Autodesk Inventor part; units mm, degrees
ref_plane "YZ Plane" through (0, 0, 0) normal (1, 0, 0) x (0, 1, 0)
ref_plane "XZ Plane" through (0, 0, 0) normal (0, 1, 0) x (-1, 0, 0)
ref_plane "XY Plane" through (0, 0, 0) normal (0, 0, 1) x (1, 0, 0)
sketch "Sketch1" plane through (0, 0, 0) normal (0, 0, 1) x (1, 0, 0)
  line L0 (0, 0) -> (164.5, 0)
  line L1 (164.5, 0) -> (164.5, 10)
  line L2 (164.5, 10) -> (0, 10)
  line L3 (0, 10) -> (0, 0)
  circle A0 centre (57, 5) radius 1.6
  circle A1 centre (99, 5) radius 1.6
  circle A2 centre (159.5, 5) radius 1.6
  circle A3 centre (147, 5) radius 1.6
  circle A4 centre (15, 5) radius 1.6
  circle A5 centre (5, 5) radius 1.6
  dimension "d1" = 10
  dimension "d2" = 90
  dimension "d4" = 3.2
  dimension "d6" = 3.2
  dimension "d7" = 3.2
  dimension "d8" = 42
  dimension "d9" = 60.5
  dimension "d26" = 3.2
  dimension "d27" = 48
  dimension "d28" = 3.2
  dimension "d29" = 42
  dimension "d32" = 15
  dimension "d33" = 5
  dimension "d61" = 3.2
  dimension "d62" = 10
  dimension "d63" = 12.5
ref_plane "Work Plane2" through (0, 0, 0) normal (0, -1, 0) x (1, 0, 0)
sketch "Sketch2" plane through (0, 0, 0) normal (0, -1, 0) x (1, 0, 0)
  circle A0 centre (52, 7) radius 1.6
  circle A1 centre (125, 7) radius 1.6
  circle A2 centre (88.5, 7) radius 1.6
  point P0 (0, 0)
  dimension "d13" = 3.2
  dimension "d15" = 3.2
  dimension "d17" = 3.2
  dimension "d18" = 36.5
  dimension "d64" = 52
  dimension "d65" = 36.5
ref_plane "Work Plane1" through (0, 0, 11) normal (0, 0, 1) x (1, 0, 0)
extrude "klocek" add sketch "Sketch1" along normal blind 11
ref_plane "Work Plane3" through (0, 0, 0) normal (0, -1, 0) x (1, 0, 0)
extrude "prowadzenie osi" cut sketch "Sketch2" against normal up to next
ref_plane "Work Plane4" through (0, 0, 0) normal (0, -1, 0) x (1, 0, 0)
sketch "Sketch7" plane through (0, 0, 0) normal (0, -1, 0) x (1, 0, 0)
  line L0 (0, 11) -> (0, 0)
  line L1 (0, 11) -> (164.5, 11)
  line L2 (0, 11) -> (40, 11)
  line L3 (40, 11) -> (0, 0)
  point P0 (0, -1.8333)
  dimension "d86" = 11
  dimension "d87" = 40
sketch "Sketch8" plane through (0, 0, 0) normal (0, -1, 0) x (1, 0, 0)
  line L0 (164.5, 0) -> (164.5, 11)
  line L1 (164.5, 11) -> (164.5, 3)
  line L2 (164.5, 11) -> (0, 11)
  line L3 (164.5, 11) -> (134.5, 11)
  line L4 (134.5, 11) -> (164.5, 3)
  point P0 (0, 0)
  point P1 (40.8333, 11)
  dimension "d80" = 8
  dimension "d81" = 30
extrude "przedni skos" cut sketch "Sketch7" against normal up to next
extrude "tylni skos" cut sketch "Sketch8" against normal up to next
ref_plane "Work Plane7" through (0, 0, 11) normal (0, 0, 1) x (1, 0, 0)
sketch "Sketch5" plane through (0, 0, 11) normal (0, 0, 1) x (1, 0, 0)
  circle A0 centre (99, 5) radius 1.6
  line L0 (95.5936, 5) -> (97.2968, 7.95)
  line L1 (97.2968, 7.95) -> (100.7032, 7.95)
  line L2 (100.7032, 7.95) -> (102.4064, 5)
  line L3 (102.4064, 5) -> (100.7032, 2.05)
  line L4 (100.7032, 2.05) -> (97.2968, 2.05)
  line L5 (97.2968, 2.05) -> (95.5936, 5)
  circle A1 centre (57, 5) radius 1.6
  line L6 (60.4064, 5) -> (58.7032, 2.05)
  line L7 (58.7032, 2.05) -> (55.2968, 2.05)
  line L8 (55.2968, 2.05) -> (53.5936, 5)
  line L9 (53.5936, 5) -> (55.2968, 7.95)
  line L10 (55.2968, 7.95) -> (58.7032, 7.95)
  line L11 (58.7032, 7.95) -> (60.4064, 5)
  point P0 (119.5, 5)
  dimension "d98" = 5.9
  dimension "d100" = 5.9
extrude "hex insert middle" cut sketch "Sketch5" against normal blind 3
ref_plane "Work Plane6" through (0, 0, 11) normal (0, 0, 1) x (1, 0, 0)
sketch "Sketch9" plane through (0, 0, 11) normal (0, 0, 1) x (1, 0, 0)
  circle A0 centre (147, 5) radius 1.6
  line L0 (150.4064, 5) -> (148.7032, 2.05)
  line L1 (148.7032, 2.05) -> (145.2968, 2.05)
  line L2 (145.2968, 2.05) -> (143.5936, 5)
  line L3 (143.5936, 5) -> (145.2968, 7.95)
  line L4 (145.2968, 7.95) -> (148.7032, 7.95)
  line L5 (148.7032, 7.95) -> (150.4064, 5)
  point P0 (0, 0)
  point P1 (153, 5)
  dimension "d99" = 5.9
extrude "hex insert rear 1" cut sketch "Sketch9" against normal blind 6
ref_plane "Work Plane5" through (0, 0, 11) normal (0, 0, 1) x (1, 0, 0)
sketch "Sketch10" plane through (0, 0, 11) normal (0, 0, 1) x (1, 0, 0)
  circle A0 centre (159.5, 5) radius 1.6
  line L0 (162.9064, 5) -> (161.2032, 2.05)
  line L1 (161.2032, 2.05) -> (157.7968, 2.05)
  line L2 (157.7968, 2.05) -> (156.0936, 5)
  line L3 (156.0936, 5) -> (157.7968, 7.95)
  line L4 (157.7968, 7.95) -> (161.2032, 7.95)
  line L5 (161.2032, 7.95) -> (162.9064, 5)
  point P0 (0, 0)
  dimension "d101" = 5.9
extrude "hex insert rear 2" cut sketch "Sketch10" against normal blind 8.5
sketch "Sketch13" plane through (0, 0, 11) normal (0, 0, 1) x (1, 0, 0)
  circle A0 centre (5, 5) radius 1.6
  line L0 (8.4064, 5) -> (6.7032, 2.05)
  line L1 (6.7032, 2.05) -> (3.2968, 2.05)
  line L2 (3.2968, 2.05) -> (1.5936, 5)
  line L3 (1.5936, 5) -> (3.2968, 7.95)
  line L4 (3.2968, 7.95) -> (6.7032, 7.95)
  line L5 (6.7032, 7.95) -> (8.4064, 5)
  point P0 (0, 0)
  dimension "d90" = 5.9
extrude "hex insert front 1" cut sketch "Sketch13" against normal through all
sketch "Sketch16" plane through (0, 0, 11) normal (0, 0, 1) x (1, 0, 0)
  circle A0 centre (15, 5) radius 1.6
  line L0 (18.4064, 5) -> (16.7032, 2.05)
  line L1 (16.7032, 2.05) -> (13.2968, 2.05)
  line L2 (13.2968, 2.05) -> (11.5936, 5)
  line L3 (11.5936, 5) -> (13.2968, 7.95)
  line L4 (13.2968, 7.95) -> (16.7032, 7.95)
  line L5 (16.7032, 7.95) -> (18.4064, 5)
  point P0 (0, 0)
  dimension "d93" = 5.9
extrude "hex insert front 2" cut sketch "Sketch16" against normal blind 9
sketch "Sketch17" plane through (0, 0, 0) normal (0, 0, -1) x (-1, 0, 0)
  line L0 (0, 10) -> (0, 0)
  line L1 (0, 0) -> (-3.2968, 0)
  line L2 (-3.2968, 0) -> (-3.2968, 10.0042)
  line L3 (-3.2968, 10.0042) -> (0, 10.0042)
  line L4 (0, 10.0042) -> (0, 0)
extrude "Extrusion20" cut sketch "Sketch17" against normal up to next
sketch "Sketch18" plane through (40, 0, 11) normal (0, -1, 0) x (1, 0, 0)
  line L0 (9.5, 0) -> (9.5, -2)
  line L1 (9.5, -2) -> (-3.5, -2)
  line L2 (-3.5, -2) -> (-3.5, 0)
  line L3 (-3.5, 0) -> (9.5, 0)
  line L4 (94.5, 0) -> (0, 0)
  circle A0 centre (12, -4) radius 1.6
  line L5 (-36.7032, -11) -> (124.5, -11)
  point P0 (-40, -11)
  dimension "d102" = 2
  dimension "d103" = 13
  dimension "d104" = 2.5
extrude "Extrusion21" cut sketch "Sketch18" against normal blind 8 contours L0 L1 L2 L3
properties part number "wheel_support_v2"
Geometry check sheet. Reference: the model listing, model coordinates, mm. A direction names the side the tool comes from. Round coordinates to 2 decimals unless told otherwise and drop trailing zeros. Loops run counter-clockwise (first coordinate to the right, second up) from the corner with the lowest first, then second, coordinate; pieces in that order, holes last. Notation, with made-up numbers: M 6,-24 L 51,-24 A10 cw 51,-9 Z; hole C 34,23 d7. An arc over 180 degrees is marked long. Return JSON: item names as keys, results as strings. Group by question number.
(1) Section check B-B, the plane x = 57. Enter the section's corners in (y, z), and give its area (3 significant figures).
(2) Set-up check for faces 3 (the face through (99, 2.05, 10)), 4 (the face through (13.4, 4.93, 0.99)), 5 (the face through (43, 4, 9)): record each of +Z, -Z, +X, -X, +Y, -Y from which the full face is reachable in a straight line by a thin tool's end or side.
(3) Go/stop test with a flat-tipped pin: pin 1 (3 mm diameter, centred on x = 57.5, y = 5, fed in from +Z). Record where the tip stops, or that it passes through.
(4) Mould release check, pull along X, two halves, no side actions. Record for faces 1 (the face through (15, 7.95, 3)), 2 (the face through (83, 5, 0)): pulls with the +X half, pulls with the -X half, needs draft (parallel to the pull), parting line crosses it, or undercut.
(5) Scan lines: line 1 along Y through (x, z) = (159.5, 1.8); line 2 along Y through (x, z) = (97.5, 10); line 3 along Z through (x, y) = (44.5, 4). Record each from-to range of solid material in increasing order. Write a range as [from, to].
(6) Section check A-A, the plane x = 125. Enter the section's corners in (y, z).
(7) Section check C-C, the plane x = 15. Enter the section's corners in (y, z) (3 decimals), and give its area (3 significant figures).
Data:
{
 "1": {"outline": "M 0,0 L 3.4,0 L 3.4,8 L 2.05,8 L 2.05,11 L 0,11 Z; M 6.6,0 L 10,0 L 10,11 L 7.95,11 L 7.95,8 L 6.6,8 Z", "area": "66.7 mm²"},
 "2": {"face 3": "+Z", "face 4": "+Z, -Z", "face 5": "+Z, -Y"},
 "3": {"pin 1": "z = 8"},
 "4": {"face 1": "undercut", "face 2": "needs draft"},
 "5": {"line 1": "[0, 3.4], [6.6, 10]", "line 2": "[0, 2.05], [7.95, 10]", "line 3": "[0, 9]"},
 "6": {"outline": "M 0,0 L 10,0 L 10,5.4 L 0,5.4 Z; M 0,8.6 L 10,8.6 L 10,11 L 0,11 Z"},
 "7": {"outline": "M 0,0 L 3.4,0 L 3.4,2 L 2.05,2 L 2.05,4.125 L 0,4.125 Z; M 6.6,0 L 10,0 L 10,4.125 L 7.95,4.125 L 7.95,2 L 6.6,2 Z", "area": "22.3 mm²"}
}
